Geometry: final body of the model. Coordinates: model frame, mm. Give positions to 0.01 mm unless a question says otherwise; leave off trailing zeros. Write each loop counter-clockwise with the first axis right and the second up, starting at its lowest first coordinate (ties: lowest second). Pieces come first, ordered by that corner, then holes. Notation, with made-up numbers: (65.5, -6) - (123.5, -6) arc R16 ccw to (123.5, 12) - close; hole circle Ø8 at (-5, 27). An arc over 180 degrees is marked (long way). One line per question, with ' | ' between items. Start each with the question number.
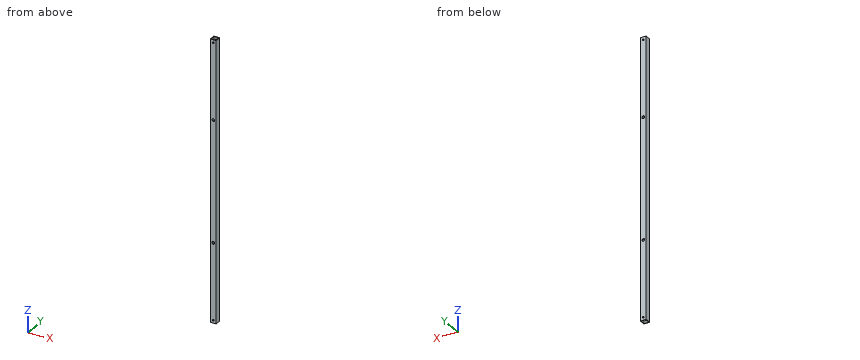
```python
from build123d import *

# Parameters (mm, degrees)
SKETCH_1_W          = 10
SKETCH_1_H          = 10
SKETCH_1_W_2        = 8
SKETCH_1_H_2        = 8
EXTRUDE_1_DEPTH     = 242.228968082
SKETCH_2_R          = 2.4
SKETCH_2_R_2        = 1.6
CUT_EXTRUDE_1_DEPTH = 243.641449423


with BuildPart() as part:
    # Sketch 1 → Extrude 1 (new body)
    with BuildSketch(Plane.XY):
        with Locations((5, 5)):
            Rectangle(SKETCH_1_W, SKETCH_1_H)
        with Locations((5, 5)):
            Rectangle(SKETCH_1_W_2, SKETCH_1_H_2, mode=Mode.SUBTRACT)
    extrude(amount=EXTRUDE_1_DEPTH)

    # Sketch 2 → Cut-Extrude 1 (cut, through all)
    with BuildSketch(Plane(origin=(0, 10, 0), x_dir=(1, 0, 0), z_dir=(0, 1, 0))):
        with Locations(Location((5, -137.228968082, 0), (0, 0, 270))):
            Circle(SKETCH_2_R)
        with Locations(Location((5, -5, 0), (0, 0, 270))):
            Circle(SKETCH_2_R_2)
    extrude(amount=-CUT_EXTRUDE_1_DEPTH, mode=Mode.SUBTRACT)

    # Mirror 1: part across plane


with BuildPart() as part_1:
    add(part.part)
    add(part.part.mirror(Plane(origin=(0, 0, 242.228968082), x_dir=(1, 0, 0), z_dir=(0, 0, -1))))


solid = part_1.part
```
1) Section B-B, the plane z = 400. Output: boundary loops of the cut face in (x, y).
2) First-contact query: pin 1 Ø4.5 at (x, z) = (5, 347.23) entering from -Y. Flat tip, straight axial feed; report the tip coordinate or a pass-through.
3) Section A-A, the plane y = 2.5. Output: boundary loops of the cut face in (x, z).
4) Section C-C, the plane x = 5. Give the number of separate pieces and of enclosed holes in the cut face, plus the area to 3 significant figures.
5) Line query: L1, parallel to Y at x = 8.5, z = 371; L2, parallel to X at y = 9.6, z = 5. Output: solid intervals per line, ascending.
Answer key:
1) outline: (0, 0) - (10, 0) - (10, 10) - (0, 10) - close; hole (1, 1) - (9, 1) - (9, 9) - (1, 9) - close
2) pin 1: through
3) outline: (0, 0) - (1, 0) - (1, 484.46) - (0, 484.46) - close; (9, 0) - (10, 0) - (10, 484.46) - (9, 484.46) - close
4) separate pieces: 10 | enclosed holes: 0 | area: 937 mm^2
5) L1: 0 to 1, 9 to 10 | L2: 0 to 3.4, 6.6 to 10
